Could you check a few things on this drawing? It's one solid part, dimensions in mm from its lowest x, y, z. A direction names the side the tool comes from. Coordinates: 2 decimals unless noted, no trailing zeros. Order: outer loops, then holes, each group sorted by start corner. A loop starts at its lowest first (then second) coordinate and runs counter-clockwise, first axis right, second up.
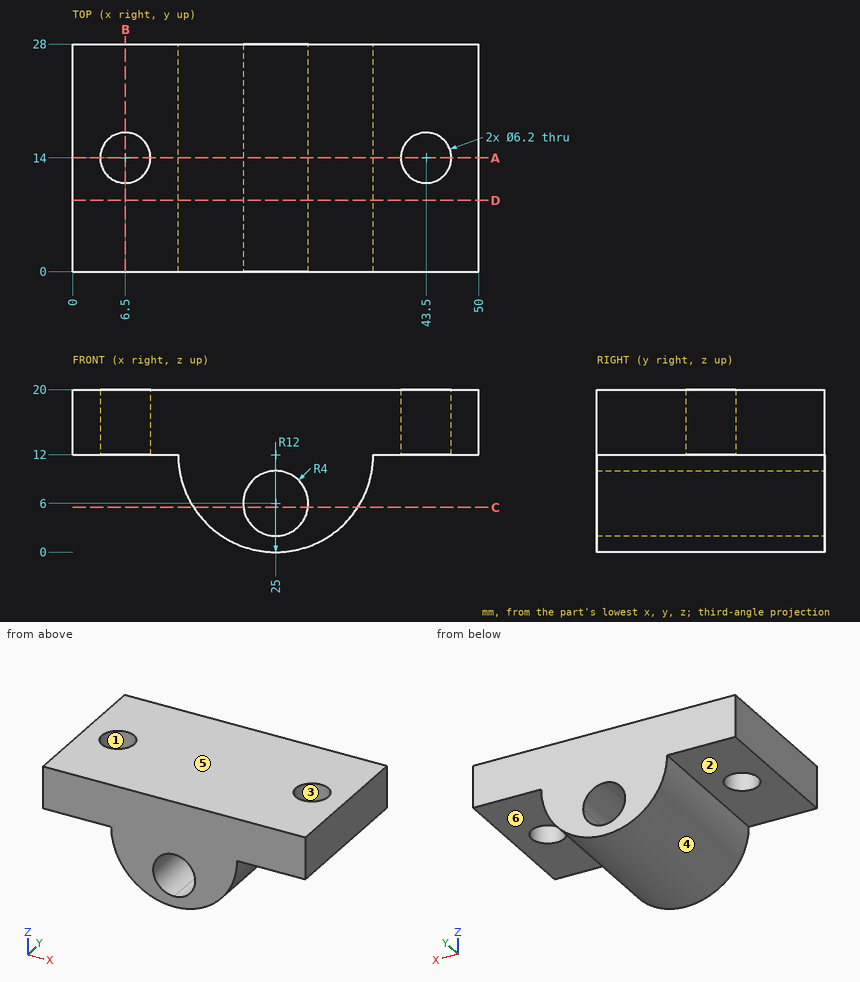
Q1. If we section it at C-C on z = 5.5: Write out the boundary of the cut face in (x, y), then the cut area to 3 significant figures.
Q2. If we section it at D-D on y = 8.75: Write out the boundary of the cut face in (x, z), then the cut area to 3 significant figures.
Q3. If we section it at A-A on y = 14: Write out the boundary of the cut face in (x, z), then the cut area to 3 significant figures.
Q4. If we section it at B-B on x = 6.5: Write out the boundary of the cut face in (y, z), then the cut area to 3 significant figures.
Q5. Will these pins go through, and if not, where does the flat tip stop? pin 1 (3.5 mm diameter, centred on x = 6.5, y = 14, fed in from -Z); pin 2 (3 mm diameter, centred on x = 31, y = 16, fed in from -Z); pin 3 (7 mm diameter, centred on x = 43.5, y = 14, fed in from +Z); pin 4 (2 mm diameter, centred on y = 3.5, z = 3, fed in from -X).
Q6. We'd pull the mould along X, two halves only. Please class the marked faces 1, 2, 3 and 4: pulls with the +X half, pulls with the -X half, needs draft (parallel to the pull), parting line crosses it, or undercut.
Q7. For the marked faces 5 and 6, which set-ups out of +Z, -Z, +X, -X, +Y, -Y let a thin tool reach every point of the face, with its end or its side?
Q8. I need wall thicknesses on L1, parallel to X at y = 15.25, z = 16.5; L2, parallel to Y at x = 6.5, z = 16.25; L3, parallel to Z at x = 40, y = 5.25. Which ranges of each line are inside material? Lowest first, please.
Reply:
1. outline: (14.91, 0) - (21.03, 0) - (21.03, 28) - (14.91, 28) - close; (28.97, 0) - (35.09, 0) - (35.09, 28) - (28.97, 28) - close
1. area: 343 mm2
2. outline: (0, 12) - (13, 12) arc R12 ccw to (37, 12) - (50, 12) - (50, 20) - (0, 20) - close; hole circle Ø8 at (25, 6)
2. area: 576 mm2
3. outline: (0, 12) - (3.4, 12) - (3.4, 20) - (0, 20) - close; (9.6, 12) - (13, 12) arc R12 ccw to (37, 12) - (40.4, 12) - (40.4, 20) - (9.6, 20) - close; (46.6, 12) - (50, 12) - (50, 20) - (46.6, 20) - close; hole circle Ø8 at (25, 6)
3. area: 477 mm2
4. outline: (0, 12) - (10.9, 12) - (10.9, 20) - (0, 20) - close; (17.1, 12) - (28, 12) - (28, 20) - (17.1, 20) - close
4. area: 174 mm2
5. pin 1: passes through
5. pin 2: stops at z = 0.88
5. pin 3: stops at z = 20
5. pin 4: stops at x = 16.06
6. face 1: undercut
6. face 2: needs draft
6. face 3: undercut
6. face 4: parting line crosses it
7. face 5: +Z, +X, -X, +Y, -Y
7. face 6: -Z, +X, +Y, -Y
8. L1: x = 0 to 3.66, 9.34 to 40.66, 46.34 to 50
8. L2: y = 0 to 10.9, 17.1 to 28
8. L3: z = 12 to 20
